```python
from build123d import *

# Parameters (mm, degrees)
F0_W            = 1000
F0_H            = 1000
F1_DEPTH        = 51
F2_SIZE         = 175
F3_R            = 50
F5_W            = 52
F5_H            = 100
F6_DEPTH        = 100
F6_COPIES_COUNT = 4
F7_R            = 410
F8_DEPTH        = 10
F9_W            = 1332.0814967155
F9_H            = 1389.9142146111
F10_DEPTH       = 10
F11_R           = 120
F12_R           = 700
F12_R_2         = 444
F13_DEPTH       = 11
F14_R           = 700
F14_R_2         = 447.5
F15_DEPTH       = 14
F16_R           = 482.5
F16_R_2         = 447.5
F17_DEPTH       = 26
F18_R           = 1
F19_R           = 419
F19_R_2         = 307.5
F20_DEPTH       = 14
F21_R           = 286.5
F22_DEPTH       = 14


# Not quite as in the source:
# - a pattern or mirror of a feature is missing from the dataset's text; its kind, count and spacing are read off the source's solid


with BuildPart() as f1:
    # F0 (on Top) → F1 (new body)
    with BuildSketch(Plane.XY):
        Rectangle(F0_W, F0_H)
    extrude(amount=F1_DEPTH)

    # F2
    f2_edges = [f1.edges().sort_by_distance(p)[0] for p in [
        (-500, -500, 25.5),
        (500, -500, 25.5),
        (500, 500, 25.5),
        (-500, 500, 25.5),
    ]]
    chamfer(f2_edges, length=F2_SIZE)

    # F3
    f3_edges = [f1.edges().sort_by_distance(p)[0] for p in [
        (-500, -325, 25.5),
        (-325, -500, 25.5),
        (325, -500, 25.5),
        (500, -325, 25.5),
        (-500, 325, 25.5),
        (500, 325, 25.5),
        (325, 500, 25.5),
        (-325, 500, 25.5),
    ]]
    fillet(f3_edges, radius=F3_R)

    # F5 (on face) → F6 (cut)
    with BuildSketch(Plane.XY.offset(51)):
        with Locations((0, 528)):
            Rectangle(F5_W, F5_H)
    f6 = extrude(amount=-F6_DEPTH, mode=Mode.SUBTRACT)

    # F6_copies: F6 ×4 about axis
    f6_copies_axis = Axis((0, 0, 0), (0, 0, 1))
    for i in range(1, F6_COPIES_COUNT):
        add(f6.rotate(f6_copies_axis, i * 360 / F6_COPIES_COUNT), mode=Mode.SUBTRACT)

    # F7 (on Top) → F8 (cut)
    with BuildSketch(Plane.XY):
        Circle(F7_R)
    extrude(amount=F8_DEPTH, mode=Mode.SUBTRACT)

    # F9 (on Top) → F10 (cut)
    with BuildSketch(Plane.XY):
        with Locations((-30.3454697132, 79.7554552555)):
            Rectangle(F9_W, F9_H)
        Polygon((473, 313.8162338159), (473, -313.8162338159), (313.8162338159, -473), (-313.8162338159, -473), (-473, -313.8162338159), (-473, 313.8162338159), (-313.8162338159, 473), (313.8162338159, 473), align=None, mode=Mode.SUBTRACT)
    extrude(amount=F10_DEPTH, mode=Mode.SUBTRACT)

    # F11
    f11_edges = [f1.edges().sort_by_distance(p)[0] for p in [
        (-313.816234, -473, 5),
        (-473, -313.816234, 5),
        (-473, 313.816234, 5),
        (-313.816234, 473, 5),
        (473, -313.816234, 5),
        (313.816234, -473, 5),
        (313.816234, 473, 5),
        (473, 313.816234, 5),
    ]]
    fillet(f11_edges, radius=F11_R)

    # F12 (on face) → F13 (cut)
    with BuildSketch(Plane.XY.offset(51)):
        Circle(F12_R)
        Circle(F12_R_2, mode=Mode.SUBTRACT)
    extrude(amount=-F13_DEPTH, mode=Mode.SUBTRACT)

    # F14 (on face) → F15 (cut)
    with BuildSketch(Plane.XY.offset(51)):
        Circle(F14_R)
        Circle(F14_R_2, mode=Mode.SUBTRACT)
    extrude(amount=-F15_DEPTH, mode=Mode.SUBTRACT)

    # F16 (on face) → F17 (cut)
    with BuildSketch(Plane.XY.offset(51)):
        Circle(F16_R)
        Circle(F16_R_2, mode=Mode.SUBTRACT)
    extrude(amount=-F17_DEPTH, mode=Mode.SUBTRACT)

    # F18
    f18_edges = [f1.edges().sort_by_distance(p)[0] for p in [
        (-341.179022, 341.179022, 25),
        (341.179022, 341.179022, 25),
        (341.179022, -341.179022, 25),
        (-341.179022, -341.179022, 25),
        (-447.5, 0, 25),
        (-444, 0, 40),
        (-447.5, 0, 40),
        (-444, 0, 51),
    ]]
    fillet(f18_edges, radius=F18_R)

    # F19 (on face) → F20 (cut)
    with BuildSketch(Plane.XY.offset(51)):
        Circle(F19_R)
        Circle(F19_R_2, mode=Mode.SUBTRACT)
    extrude(amount=-F20_DEPTH, mode=Mode.SUBTRACT)

    # F21 (on face) → F22 (cut)
    with BuildSketch(Plane.XY.offset(51)):
        Circle(F21_R)
    extrude(amount=-F22_DEPTH, mode=Mode.SUBTRACT)


solid = f1.part
```
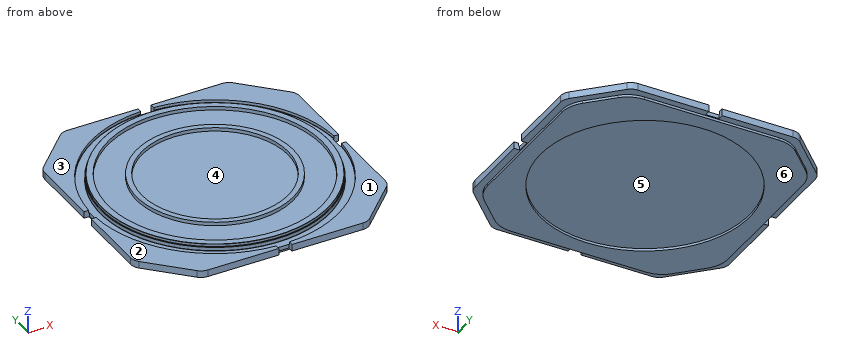
The listing builds one solid part. Answer for the finished solid, in the listing's coordinates (mm). Face numbers are marked on the shaded views. A direction names the side the tool comes from. Coordinates: 2 decimals unless noted, no trailing zeros. Return JSON: item names as keys, results as strings. Group by question number.
(1) Find the intervals of material crossed by probe 1 along Y at (x, z) = (0, 44); probe 2 along X at (y, z) = (109, 27); probe 3 along X at (y, z) = (47.5, 42.5), in increasing order. Write a range as from..to.
(2) Determine the mould class of the marked faces 5 and 6 for opening direction Y: released by +Y, released by -Y, zero draft, split by the parting line, or undercut.
(3) Given pin 1 Ø3 at (x, z) = (-16.5, 4) entering from -Y; pin 2 Ø10 at (x, y) = (193.5, 191) entering from -Z; pin 3 Ø6.5 at (y, z) = (485, 20.5) entering from +X, each flat-ended and moving along its own axis, determine where each tip first touches the part or whether it passes through.
(4) Which of the six approach directions +Z, -Z, +X, -X, +Y, -Y give full straight-line access (tool end or side, diameter ignored) to the marked faces 1, 2, 3 and 4?
The answers:
{
 "1": {"probe 1": "y = -444..-419, -307.5..-286.5, 286.5..307.5, 419..444", "probe 2": "x = -500..-470.03, -434.02..434.02, 470.03..500", "probe 3": "x = -441.45..-416.3, -303.81..-282.53, 282.53..303.81, 416.3..441.45"},
 "2": {"face 5": "undercut", "face 6": "zero draft"},
 "3": {"pin 1": "stops at y = -473", "pin 2": "stops at z = 10", "pin 3": "stops at x = 343.25"},
 "4": {"face 1": "+Z, +X, -Y", "face 2": "+Z, -X, -Y", "face 3": "+Z, -X, +Y", "face 4": "+Z"}
}
